```python
from build123d import *

# Parameters (mm, degrees)
RESSALTO_EXTRUS_O1_START = -10.4
RESSALTO_EXTRUS_O1_DEPTH = 10.4
PADR_OCIRCULAR1_COUNT    = 15
ESBO_O3_R                = 3.3
CORTE_EXTRUS_O1_DEPTH    = 22
CORTE_EXTRUS_O4_DEPTH    = 20


with BuildPart() as part:
    # Esboço1 → Revolução1 (revolve)
    with BuildSketch(Plane.XY, mode=Mode.PRIVATE) as revolu_o1_sk:
        Polygon((0, 0), (0, 39.4), (5.9, 39.4), (5.9, 33.4), (7.5, 33.4), (7.5, 32.4), (9.374, 32.4), (9.374, 22), (8.47, 22), (8.47, 18.51), (9.9, 18.51), (9.9, 17.01), (8.47, 15.58), (8.47, 0), align=None)
    revolve(revolu_o1_sk.sketch.rotate(Axis((0, 0, 0), (0, 1, 0)), 90), axis=Axis((0, 0, 0), (0, 1, 0)))

    # Esboço2 → Ressalto-extrusão1 (add)
    with BuildSketch(Plane(origin=(0, 32.4, 0), x_dir=(1, 0, 0), z_dir=(0, 1, 0)).offset(RESSALTO_EXTRUS_O1_START)):
        with BuildLine():
            Line((-0.337, 12.746), (0.337, 12.746))
            ThreePointArc((0.337, 12.746), (1.105703178, 11.108702403), (1.167644885, 9.300993572))
            ThreePointArc((1.167644885, 9.300993572), (0, 9.374), (-1.167644885, 9.300993572))
            ThreePointArc((-1.167644885, 9.300993572), (-1.105703178, 11.108702403), (-0.337, 12.746))
        make_face()
    ressalto_extrus_o1 = extrude(amount=RESSALTO_EXTRUS_O1_DEPTH)

    # PadrãoCircular1: Ressalto-extrusão1 ×15 about axis
    padr_ocircular1_axis = Axis((0, 0, 0), (0, 1, 0))
    for i in range(1, PADR_OCIRCULAR1_COUNT):
        add(ressalto_extrus_o1.rotate(padr_ocircular1_axis, i * 360 / PADR_OCIRCULAR1_COUNT))

    # Esboço3 → Corte-extrusão1 (cut)
    with BuildSketch(Plane.XZ):
        with Locations(Location((0, 0, 0), (0, 0, 270))):
            Circle(ESBO_O3_R)
    extrude(amount=-CORTE_EXTRUS_O1_DEPTH, mode=Mode.SUBTRACT)

    # Esboço7 → Corte-extrusão4 (cut, symmetric)
    with BuildSketch(Plane(origin=(0, 0, 0), x_dir=(0, 0, -1), z_dir=(1, 0, 0))):
        with BuildLine():
            Line((-2.6, 5.5), (-2.6, 3.5))
            ThreePointArc((-2.6, 3.5), (0, 0.9), (2.6, 3.5))
            Line((2.6, 3.5), (2.6, 5.5))
            ThreePointArc((2.6, 5.5), (0, 8.1), (-2.6, 5.5))
        make_face()
    extrude(amount=CORTE_EXTRUS_O4_DEPTH, both=True, mode=Mode.SUBTRACT)


solid = part.part
```
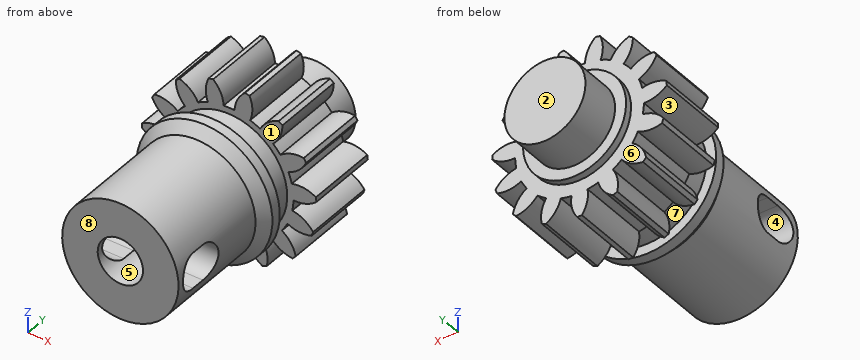
CAD build for the part. Positions are in the model's coordinates, mm. Face numbers are marked on the shaded views. A direction names the side the tool comes from. Coordinates: 2 decimals unless noted, no trailing zeros. Order: outer loops, then holes, each group sorted by start corner. A loop starts at its lowest first (then second) coordinate and runs counter-clockwise, first axis right, second up. Notation, with made-up numbers: (14, 89) - (47, 89) arc R15 cw to (47, 93) - close; hole circle Ø5 at (71.5, 4). An arc over 180 degrees is marked (long way). Use a Markdown table: item, result. Add a question column.
(1) Flat gauge pins, fed straight in: pin 1 (5 mm diameter, centred on x = 7, y = 29, fed in from -Z); pin 2 (0.6 mm diameter, centred on x = -5, y = 4.5, fed in from -Z); pin 3 (4 mm diameter, centred on y = 23, z = 5, fed in from -X). Where does each tip first touch, or does it go through?
(2) Drill centre lines: line 1 along X through (y, z) = (12.5, 0); line 2 along X through (y, z) = (32, 9.5); line 3 along Y through (x, z) = (3.5, -0.25). Where is each one in solid material? Low to high. Write a range as [from, to].
(3) Pull direction Y, two halves, no side cores. Call the marked faces 1, 2 and 3: +Y half, -Y half, draft (parallel to the pull), parting line (faces both ways), or undercut.
(4) Saw through at A-A (y = 17.5). Give the cut face in (x, z).
(5) Which spindle directions (+Z, -Z, +X, -X, +Y, -Y) get a long thin tool onto all of the face, cutting with end or side? Do the marked faces 4, 5, 6, 7 and 8. Say none if no direction does.
Solved:
| question | item | result |
|---|---|---|
| 1 | pin 1 | stops at z = -11.78 |
| 1 | pin 2 | stops at z = -7.05 |
| 1 | pin 3 | stops at x = -11.21 |
| 2 | line 1 | x = [-8.47, -3.3], [3.3, 8.47] |
| 2 | line 2 | x = [-7.73, -5.48], [-3.28, -0.8], [0.8, 3.28], [5.48, 7.73] |
| 2 | line 3 | y = [0, 0.91], [8.09, 39.4] |
| 3 | face 1 | undercut |
| 3 | face 2 | +Y half |
| 3 | face 3 | draft |
| 4 | outline | circle Ø19.8 at (0, 0); hole circle Ø6.6 at (0, 0) |
| 5 | face 4 | +X, -X |
| 5 | face 5 | -Y |
| 5 | face 6 | +Y |
| 5 | face 7 | none |
| 5 | face 8 | +Z, -Z, +X, -X, -Y |
